Geometry: final body of the model. Coordinates: model frame, mm. Give positions to 0.01 mm unless a question says otherwise; leave off trailing zeros. Loops run counter-clockwise (first coordinate to the right, second up) from the corner with the lowest first, then second, coordinate; pieces in that order, holes last. Notation, with made-up numbers: (45.25, 20.5) - (62.25, 20.5) arc R22 ccw to (62.25, 28.5) - close; hole circle Ø1 at (-30.75, 12). An arc over 180 degrees is marked (long way). Use CSV: the item, a comma, the result in double quotes. Start each with the question number.
```python
from build123d import *

# Parameters (mm, degrees)
MODEL_R                 = 1.5
SALIENTE_EXTRUIR1_DEPTH = 1


with BuildPart() as part:
    # Model → Saliente-Extruir1 (new body)
    with BuildSketch(Plane.XY):
        with BuildLine():
            Line((147.399890085, 168.7618816), (216.149890085, 168.7618816))
            ThreePointArc((216.149890085, 168.7618816), (219.3318706, 170.079901084), (220.649890085, 173.2618816))
            Line((220.649890085, 173.2618816), (220.649890085, 236.2618816))
            ThreePointArc((220.649890085, 236.2618816), (218.74210805, 239.940251622), (214.636376298, 240.499720202))
            Line((214.636376298, 240.499720202), (88.636376298, 195.499720202))
            ThreePointArc((88.636376298, 195.499720202), (86.471520063, 193.854099565), (85.649890085, 191.2618816))
            Line((85.649890085, 191.2618816), (85.649890085, 176.3868816))
            ThreePointArc((85.649890085, 176.3868816), (86.089229913, 175.326221428), (87.149890085, 174.8868816))
            Line((87.149890085, 174.8868816), (92.649890085, 174.8868816))
            ThreePointArc((92.649890085, 174.8868816), (93.180220171, 174.667211686), (93.399890085, 174.1368816))
            Line((93.399890085, 174.1368816), (93.399890085, 168.7618816))
            Line((93.399890085, 168.7618816), (140.899890085, 168.7618816))
            Line((140.899890085, 168.7618816), (140.899890085, 174.1368816))
            ThreePointArc((140.899890085, 174.1368816), (141.119559999, 174.667211686), (141.649890085, 174.8868816))
            Line((141.649890085, 174.8868816), (146.649890085, 174.8868816))
            ThreePointArc((146.649890085, 174.8868816), (147.180220171, 174.667211686), (147.399890085, 174.1368816))
            Line((147.399890085, 174.1368816), (147.399890085, 168.7618816))
        make_face()
        with Locations((99.149890085, 173.2618816)):
            Circle(MODEL_R, mode=Mode.SUBTRACT)
        with Locations((135.149890085, 173.2618816)):
            Circle(MODEL_R, mode=Mode.SUBTRACT)
    extrude(amount=SALIENTE_EXTRUIR1_DEPTH)


solid = part.part
```
Item 1: Pin query (flat end, axial travel): pin 1 Ø5 at (x, y) = (99.15, 173.26) entering from +Z; pin 2 Ø0.5 at (x, z) = (91, 0.5) entering from -Y. Return the tip coordinate at first contact, or that it passes through.
Item 2: Section C-C (x = 200). Output: boundary loops of the cut face in (y, z).
Item 3: Mould query, pull axis X, two halves, no side actions, for faces 1 (the cylindrical face through (134.82, 171.8, 0.49)), 2 (the flat face through (152.518, 218.315, 0.493)), 3 (the cylindrical face through (98.82, 171.8, 0.49)), 4 (the flat face through (167, 197, 0)). Classes: pulls with the +X half, pulls with the -X half, needs draft (parallel to the pull), parting line crosses it, or undercut.
Item 4: Section B-B (y = 217.5). Output: boundary loops of the cut face in (x, z), plus the area to 3 significant figures.
Item 5: Section A-A (z = 0.65). Output: boundary loops of the cut face in (x, y), plus the area to 3 significant figures.
Item 6: Ray query, probe 1 along Y at (x, z) = (99, 0.45); probe 2 along Y at (x, z) = (187.5, 0.45); probe 3 along Y at (x, z) = (146, 0.5). Return the intervals inside material, ascending.
Outcome:
1,pin 1,"stops at z = 1"
1,pin 2,"stops at y = 174.89"
2,outline,"(168.76, 0) - (235.27, 0) - (235.27, 1) - (168.76, 1) - close"
3,face 1,"undercut"
3,face 2,"pulls with the -X half"
3,face 3,"undercut"
3,face 4,"needs draft"
4,outline,"(150.24, 0) - (220.65, 0) - (220.65, 1) - (150.24, 1) - close"
4,area,"70.4 mm2"
5,outline,"(85.65, 176.39) arc R1.5 ccw to (87.15, 174.89) - (92.65, 174.89) arc R0.75 cw to (93.4, 174.14) - (93.4, 168.76) - (140.9, 168.76) - (140.9, 174.14) arc R0.75 cw to (141.65, 174.89) - (146.65, 174.89) arc R0.75 cw to (147.4, 174.14) - (147.4, 168.76) - (216.15, 168.76) arc R4.5 ccw to (220.65, 173.26) - (220.65, 236.26) arc R4.5 ccw to (214.64, 240.5) - (88.64, 195.5) arc R4.5 ccw to (85.65, 191.26) - close; hole circle Ø3 at (99.15, 173.26); hole circle Ø3 at (135.15, 173.26)"
5,area,"6,600 mm2"
6,probe 1,"y = 168.76 to 171.77, 174.75 to 199.2"
6,probe 2,"y = 168.76 to 230.81"
6,probe 3,"y = 174.89 to 215.99"
